Input: part model. Units: mm. Frame: model coordinates. Give positions to 0.01 mm unless a question says otherwise; leave off trailing zeros. Write each loop counter-clockwise with the first axis right and the second up, starting at its lowest first coordinate (ties: lowest second). Pieces come first, ordered by that corner, then holes.
```python
from build123d import *

# Parameters (mm, degrees)
SKETCH1_R           = 2
BOSS_EXTRUDE1_DEPTH = 3.5
FILLET1_R           = 0.5


with BuildPart() as part:
    # Sketch1 → Boss-Extrude1 (new body)
    with BuildSketch(Plane.XY):
        Polygon((-2.8145825622994267, 1.625000000000001), (-1.8763883748662844, 3.25), (0, 3.2500000000000004), (1.8763883748662837, 3.25), (2.8145825622994254, 1.6249999999999996), (3.752776749732567, -3.3e-16), (2.814582562299426, -1.6249999999999998), (1.876388374866284, -3.25), (0, -3.2500000000000004), (-1.876388374866284, -3.25), (-2.814582562299426, -1.6249999999999993), (-3.752776749732568, 8.7e-16), align=None)
        Circle(SKETCH1_R, mode=Mode.SUBTRACT)
    extrude(amount=BOSS_EXTRUDE1_DEPTH)

    # Fillet1
    fillet1_edges = [part.edges().sort_by_distance(p)[0] for p in [
        (-2.8145825622994263, 1.6250000000000004, 0),
        (-4.4e-16, 3.25, 0),
        (2.8145825622994254, 1.625, 0),
        (2.8145825622994254, -1.6250000000000002, 0),
        (0, -3.25, 3.5),
        (0, -3.25, 0),
        (-2.814582562299426, -1.6249999999999996, 0),
        (2.8145825622994254, -1.625, 3.5),
        (2.8145825622994254, 1.6249999999999998, 3.5),
        (-2.2e-16, 3.25, 3.5),
        (-2.8145825622994263, 1.6250000000000004, 3.5),
        (-2.814582562299426, -1.6249999999999996, 3.5),
    ]]
    fillet(fillet1_edges, radius=FILLET1_R)


solid = part.part
```
Q1. Section C-C, the plane z = 3.15. Return the cut outline in (x, y).
Q2. Section D-D, the plane x = 1.25. Return the cut outline in (y, z), then the cut area to 3 significant figures.
Q3. Mould query, pull axis X, two halves, no side actions, for faces 1 (the cylindrical face through (2.704, -1.531, 0.15)), 2 (the flat face through (0, -3.25, 2)), 3 (the cylindrical face through (0, -2, 2)), 4 (the cylindrical face through (-2.704, 1.531, 3.35)). Classes: +X half, -X half, draft (parallel to the pull), parting line (faces both ways), or undercut.
Q4. Section A-A, the plane x = 0. Return the cut outline in (y, z).
Q5. Material intervals for line 1 along Y through (x, z) = (0, 1.2); line 2 along X through (y, z) = (1.5, 2.5); line 3 along Y through (x, z) = (0, 3.2), sorted ascending.
Q6. Section B-B, the plane z = 1.9. Return the cut outline in (x, y), then the cut area to 3 significant figures.
Solutions:
1. outline: (-3.73, 0) - (-1.86, -3.23) - (1.86, -3.23) - (3.73, 0) - (1.86, 3.23) - (-1.86, 3.23) - close; hole circle Ø4 at (0, 0)
2. outline: (-3.25, 0.5) arc R0.5 ccw to (-2.75, 0) - (-1.56, 0) - (-1.56, 3.5) - (-2.75, 3.5) arc R0.5 ccw to (-3.25, 3) - close; (1.56, 0) - (2.75, 0) arc R0.5 ccw to (3.25, 0.5) - (3.25, 3) arc R0.5 ccw to (2.75, 3.5) - (1.56, 3.5) - close
2. area: 11.6 mm2
3. face 1: +X half
3. face 2: draft
3. face 3: undercut
3. face 4: -X half
4. outline: (-3.25, 0.5) arc R0.5 ccw to (-2.75, 0) - (-2, 0) - (-2, 3.5) - (-2.75, 3.5) arc R0.5 ccw to (-3.25, 3) - close; (2, 0) - (2.75, 0) arc R0.5 ccw to (3.25, 0.5) - (3.25, 3) arc R0.5 ccw to (2.75, 3.5) - (2, 3.5) - close
5. line 1: y = -3.25 to -2, 2 to 3.25
5. line 2: x = -2.89 to -1.32, 1.32 to 2.89
5. line 3: y = -3.21 to -2, 2 to 3.21
6. outline: (-3.75, 0) - (-1.88, -3.25) - (1.88, -3.25) - (3.75, 0) - (1.88, 3.25) - (-1.88, 3.25) - close; hole circle Ø4 at (0, 0)
6. area: 24.0 mm2
